Geometry check sheet. Reference: drawing and pictorial views, mm from the part's lowest x, y, z. A direction names the side the tool comes from. Coordinates: 2 decimals unless noted, no trailing zeros. Order: outer loops, then holes, each group sorted by start corner. A loop starts at its lowest first (then second) coordinate and runs counter-clockwise, first axis right, second up. Notation, with made-up numbers: M -22.5,13 L -14.5,13 A23 cw -14.5,45 Z; hole C 9.25,-2 d11. An arc over 180 degrees is marked long. Return JSON: item names as keys, results as strings.
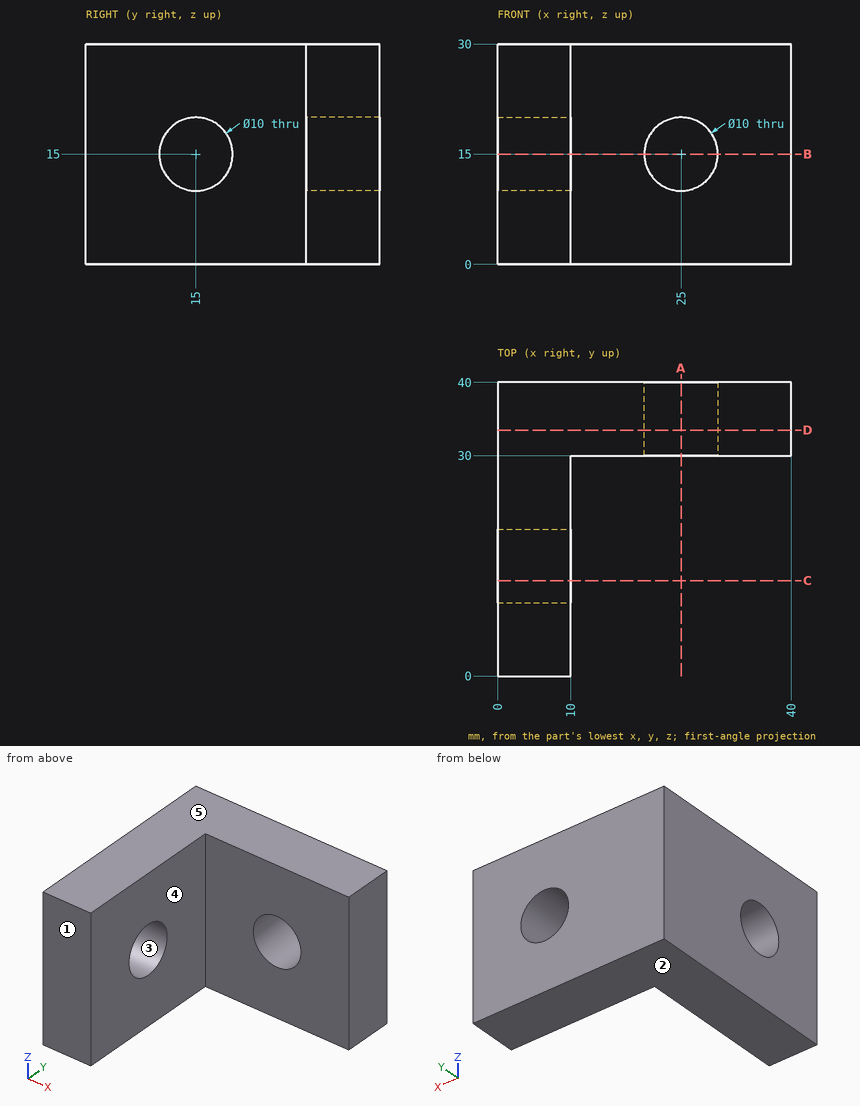
Q1. Cross-section at D-D, the plane y = 33.5. Record the boundary of the cut face in (x, z), and give its area (3 significant figures).
Values:
{"outline": "M 0,0 L 40,0 L 40,30 L 0,30 Z; hole C 25,15 d10", "area": "1,120 mm^2"}
Q2. Cross-section at A-A, the plane x = 25. Record the boundary of the cut face in (y, z).
Values:
{"outline": "M 30,0 L 40,0 L 40,10 L 30,10 Z; M 30,20 L 40,20 L 40,30 L 30,30 Z"}
Q3. Material ranges on line 1 along Z through (x, y) = (25, 34); line 2 along X through (y, z) = (36, 15); line 3 along X through (y, z) = (6, 27.25), recorded low to high.
Values:
{"line 1": "0 to 10, 20 to 30", "line 2": "0 to 20, 30 to 40", "line 3": "0 to 10"}
Q4. Cross-section at B-B, the plane z = 15. Record the boundary of the cut face in (x, y).
Values:
{"outline": "M 0,0 L 10,0 L 10,10 L 0,10 Z; M 0,20 L 10,20 L 10,30 L 20,30 L 20,40 L 0,40 Z; M 30,30 L 40,30 L 40,40 L 30,40 Z"}
Q5. Cross-section at C-C, the plane y = 13. Record the boundary of the cut face in (x, z), and give its area (3 significant figures).
Values:
{"outline": "M 0,0 L 10,0 L 10,10.42 L 0,10.42 Z; M 0,19.58 L 10,19.58 L 10,30 L 0,30 Z", "area": "208 mm^2"}
Q6. Tool access check on the marked faces 4 and 5. Record the directions out of +Z, -Z, +X, -X, +Y, -Y that give a thin tool (end or side, any length) a straight path to the whole face; none if there is none.
Values:
{"face 4": "+Z, -Z, +X, -Y", "face 5": "+Z, +X, -X, +Y, -Y"}
Q7. Go/stop test with flat-tipped pins: pin 1 (3 mm diameter, centred on y = 11.5, z = 21.5, fed in from +X); pin 2 (2 mm diameter, centred on x = 13.5, z = 15, fed in from -Y). Record where each tip stops, or that it passes through.
Values:
{"pin 1": "x = 10", "pin 2": "y = 30"}
Q8. Draft check along Z on the marked faces 1, 2 and 3. Enter one of: pulls with the +Z half, pulls with the -Z half, needs draft (parallel to the pull), parting line crosses it, or undercut.
Values:
{"face 1": "needs draft", "face 2": "pulls with the -Z half", "face 3": "undercut"}
